Work out the finished part from the listing and answer in its coordinate system (mm). A direction names the side the tool comes from. Round coordinates to 2 decimals unless told otherwise and drop trailing zeros. Order: outer loops, then holes, each group sorted by start corner. A loop starts at its lowest first (then second) coordinate and runs counter-clockwise, first axis right, second up. Notation, with made-up numbers: (7.25, 69) - (51.25, 69) arc R29 cw to (51.25, 93) - close; hole circle Ø9 at (55.5, 31). An arc over 180 degrees is marked (long way). Put each result on its own line as item: value.
```python
from build123d import *

# Parameters (mm, degrees)
F0_R     = 7
F1_DEPTH = 28.8
F2_DEPTH = 10
F3_DEPTH = 10
F4_R     = 3.9
F5_DEPTH = 32.001
F6_W     = 30
F6_H     = 12
F7_DEPTH = 50


with BuildPart() as f1:
    # F0 (on Top) → F1 (new body)
    with BuildSketch(Plane.XY):
        with BuildLine():
            Line((57.36, 0), (57.36, -12))
            Line((57.36, -12), (200, -12))
            Line((200, -12), (200, -4))
            ThreePointArc((200, -4), (198.828427, -1.171573), (196, 0))
            Line((196, 0), (77, 0))
            Line((77, 0), (57.36, 0))
        make_face()
        with BuildLine():
            ThreePointArc((11.87692, 1.714286), (-9.071147, 7.855844), (0, -12))
            Line((0, -12), (47.36, -12))
            Line((47.36, -12), (42.36, 0))
            Line((42.36, 0), (13.856406, 0))
            ThreePointArc((13.856406, 0), (12.547099, 0.488142), (11.87692, 1.714286))
        make_face()
        Circle(F0_R, mode=Mode.SUBTRACT)
        Polygon((42.36, 0), (47.36, -12), (57.36, -12), (57.36, 0), align=None)
    extrude(amount=-F1_DEPTH)

    # F0 (on Top) → F2 (join)
    with BuildSketch(Plane.XY):
        with BuildLine():
            ThreePointArc((65, 20), (63.024853, 9.295266), (57.36, 0))
            Line((57.36, 0), (77, 0))
            ThreePointArc((77, 0), (75.585786, 0.585786), (75, 2))
            Line((75, 2), (75, 16))
            ThreePointArc((75, 16), (73.828427, 18.828427), (71, 20))
            Line((71, 20), (65, 20))
        make_face()
    extrude(amount=-F2_DEPTH)

    # F0 (on Top) → F3 (cut)
    with BuildSketch(Plane.XY):
        Polygon((42.36, 0), (47.36, -12), (57.36, -12), (57.36, 0), align=None)
    extrude(amount=-F3_DEPTH, mode=Mode.SUBTRACT)

    # F4 (on face) → F5 (cut, through all)
    with BuildSketch(Plane.XZ.offset(12)):
        with Locations((177, -19.4)):
            Circle(F4_R)
    extrude(amount=-F5_DEPTH, mode=Mode.SUBTRACT)

    # F6 (on Front) → F7 (cut, symmetric)
    with BuildSketch(Plane.XZ):
        with Locations((-0.769001, -14.4)):
            Rectangle(F6_W, F6_H)
    extrude(amount=F7_DEPTH, both=True, mode=Mode.SUBTRACT)


solid = f1.part
```
1) A cutting plane is placed at C-C on z = -17.5. Write down the section's boundary in (x, y).
Findings below:
outline: (14.23, -12) - (173.59, -12) - (173.59, 0) - (14.23, 0) - close; (180.41, -12) - (200, -12) - (200, -4) arc R4 ccw to (196, 0) - (180.41, 0) - close
2) Straight lines are drawn through the part: L1, parallel to Y at x = 0, z = -26; L2, parallel to Z at x = 177, y = -9.25; L3, parallel to Z at x = 6.5, y = 7. For each, find the intervals that lie inside material, in ascending order. Write a range as from..to.
Findings below:
L1: y = -12..-7, 7..12
L2: z = -28.8..-23.3, -15.5..0
L3: z = -28.8..-20.4, -8.4..0
3) A cutting plane is placed at A-A on z = -3. Write down the section's boundary in (x, y), then the cut area to 3 significant figures.
Findings below:
outline: (0, -12) - (47.36, -12) - (42.36, 0) - (13.86, 0) arc R2 cw to (11.88, 1.71) arc R12 ccw (long way) to start; (57.36, -12) - (200, -12) - (200, -4) arc R4 ccw to (196, 0) - (77, 0) arc R2 cw to (75, 2) - (75, 16) arc R4 ccw to (71, 20) - (65, 20) arc R30 cw to (57.36, 0) - close; hole circle Ø14 at (0, 0)
area: 2,680 mm2
4) For a pull along Z with two mould halves and no side action, classify faces 4 (the flat face through (112, -6, 0)), 5 (the cylindrical face through (198.859, -1.203, -14.198)), 6 (the flat face through (7, -3, -20.4)) as pulls with the +Z half, pulls with the -Z half, needs draft (parallel to the pull), parting line crosses it, or undercut.
Findings below:
face 4: pulls with the +Z half
face 5: needs draft
face 6: undercut
5) A cutting plane is placed at B-B on x = 177. Write down the section's boundary in (y, z).
Findings below:
outline: (-12, -28.8) - (0, -28.8) - (0, -23.3) - (-12, -23.3) - close; (-12, -15.5) - (0, -15.5) - (0, 0) - (-12, 0) - close
6) A cutting plane is placed at D-D on x = 38. Write down the section's boundary in (y, z), then the cut area to 3 significant figures.
Findings below:
outline: (-12, -28.8) - (0, -28.8) - (0, 0) - (-12, 0) - close
area: 346 mm2
7) Given pin 1 Ø2 at (x, z) = (59.5, -5) entering from +Y; pin 2 Ø3.5 at (y, z) = (-5, -16.5) entering from -X; pin 3 Ø10 at (x, y) = (66.5, 9) entering from -Z, each flat-ended and moving along its own axis, determine where each tip first touches the part or whether it passes through.
Findings below:
pin 1: stops at y = 4.2
pin 2: stops at x = 14.23
pin 3: stops at z = -10
8) For faces 1 (the flat face through (51, -6, -10)), 2 (the flat face through (14.231, -6, -14)), 3 (the flat face through (75, 9, -5)), determine the directions among +Z, -Z, +X, -X, +Y, -Y from which every point of the face is accessible in a straight line to the end or side of a thin tool.
Findings below:
face 1: +Z, +Y
face 2: -X, +Y, -Y
face 3: +Z, -Z, +X, +Y
